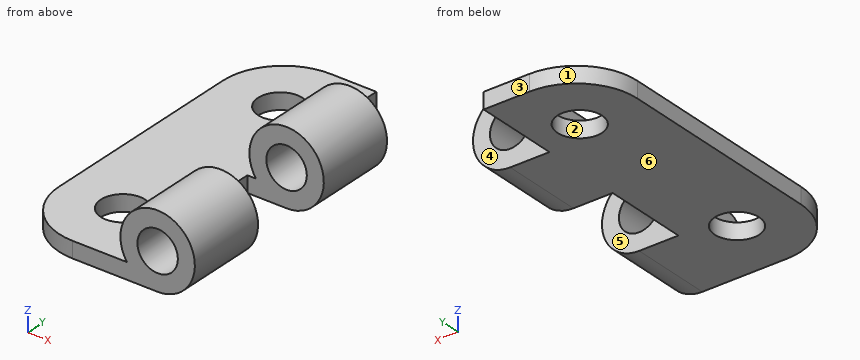
Autodesk Inventor part; units mm, degrees
ref_plane "l_pin_XY" through (0, 0, 0) normal (0, 1, 0) x (1, 0, 0)
ref_plane "l_pin_YZ" through (0, 0, 0) normal (1, 0, 0) x (0, 0, -1)
ref_plane "l_pin_ZX" through (0, 0, 0) normal (0, 0, -1) x (0, 1, 0)
sketch "Sketch_1" plane through (0, 0, 0) normal (0, 0, 1) x (1, 0, 0)
  line L0 (0, -20.5) -> (0, 20.5)
  line L1 (0, 20.5) -> (4.6, 20.5)
  line L2 (4.6, 20.5) -> (4.6, -20.5)
  line L3 (4.6, -20.5) -> (0, -20.5)
  line L4 (0, -20.5) -> (0, 20.5)
revolve "Revolution1" add sketch "Sketch_1" angle 360 about axis through (0, -20.5, 0) along (0, -1, 0)
sketch "Sketch_2" plane through (0, 0, -4.6) normal (0, 0, 1) x (1, 0, 0)
  line L0 (-18, 13) -> (-18, -13)
  arc A0 (-18, -13) -> (-10.5, -20.5) centre (-10.5, -13) ccw
  line L1 (-10.5, -20.5) -> (0, -20.5)
  line L2 (0, -20.5) -> (0, 20.5)
  line L3 (0, 20.5) -> (-10.5, 20.5)
  arc A1 (-10.5, 20.5) -> (-18, 13) centre (-10.5, 13) ccw
extrude "Extrusion1" add sketch "Sketch_2" along normal blind 2
sketch "Sketch_3" plane through (0, 0, 0) normal (0, 0, 1) x (1, 0, 0)
  line L0 (-41, 41) -> (-41, -41)
  line L1 (-41, -41) -> (41, -41)
  line L2 (41, -41) -> (41, 41)
  line L3 (41, 41) -> (-41, 41)
  line L4 (-18, 20.5) -> (-18, -20.5)
  line L5 (-18, -20.5) -> (4.6, -20.5)
  line L6 (4.6, -20.5) -> (4.6, -10.45)
  line L7 (4.6, -10.45) -> (-4.85, -10.45)
  line L8 (-4.85, -10.45) -> (-4.85, 0)
  line L9 (-4.85, 0) -> (4.6, 0)
  line L10 (4.6, 0) -> (4.6, 10.05)
  line L11 (4.6, 10.05) -> (-4.85, 10.05)
  line L12 (-4.85, 10.05) -> (-4.85, 20.5)
  line L13 (-4.85, 20.5) -> (-18, 20.5)
extrude "Extrusion2" cut sketch "Sketch_3" along normal mid plane 82
sketch "Sketch_4" plane through (0, 0, 0) normal (0, 0, 1) x (1, 0, 0)
  line L0 (0, -20.5) -> (0, 20.5)
  line L1 (0, 20.5) -> (2.5, 20.5)
  line L2 (2.5, 20.5) -> (2.5, -20.5)
  line L3 (2.5, -20.5) -> (0, -20.5)
  line L4 (0, -20.5) -> (0, 20.5)
revolve "Revolution2" cut sketch "Sketch_4" angle 360 about axis through (0, -20.5, 0) along (0, -1, 0)
sketch "Sketch_11" plane through (0, 12.5, 0) normal (0, 1, 0) x (1, 0, 0)
  line L0 (-10.5, 2.6) -> (-10.5, 4.6)
  line L1 (-10.5, 4.6) -> (-7.75, 4.6)
  line L2 (-7.75, 4.6) -> (-7.75, 2.6)
  line L3 (-7.75, 2.6) -> (-10.5, 2.6)
  line L4 (-10.5, 2.6) -> (-10.5, 4.6)
revolve "Revolution3" cut sketch "Sketch_11" angle 360 about axis through (-10.5, 12.5, -2.6) along (0, 0, 1)
sketch "Sketch_5" plane through (0, -12.5, 0) normal (0, 1, 0) x (1, 0, 0)
  line L0 (-10.5, 2.6) -> (-10.5, 4.6)
  line L1 (-10.5, 4.6) -> (-7.75, 4.6)
  line L2 (-7.75, 4.6) -> (-7.75, 2.6)
  line L3 (-7.75, 2.6) -> (-10.5, 2.6)
  line L4 (-10.5, 2.6) -> (-10.5, 4.6)
revolve "Revolution4" cut sketch "Sketch_5" angle 360 about axis through (-10.5, -12.5, -2.6) along (0, 0, 1)
ref_plane "l_pin_XY" through (0, 0, 0) normal (0, 1, 0) x (1, 0, 0)
ref_plane "l_pin_YZ" through (0, 0, 0) normal (1, 0, 0) x (0, 0, -1)
ref_plane "l_pin_ZX" through (0, 0, 0) normal (0, 0, -1) x (0, 1, 0)
ref_plane "hole1l_to_bolt_XY" through (-10.5, 12.5, -2.6) normal (0, 0, 1) x (1, 0, 0)
ref_plane "hole1l_to_bolt_YZ" through (-10.5, 12.5, -2.6) normal (1, 0, 0) x (0, 1, 0)
ref_plane "hole1l_to_bolt_ZX" through (-10.5, 12.5, -2.6) normal (0, 1, 0) x (0, 0, 1)
ref_plane "hole2l_to_bolt_XY" through (-10.5, -12.5, -2.6) normal (0, 0, 1) x (1, 0, 0)
ref_plane "hole2l_to_bolt_YZ" through (-10.5, -12.5, -2.6) normal (1, 0, 0) x (0, 1, 0)
ref_plane "hole2l_to_bolt_ZX" through (-10.5, -12.5, -2.6) normal (0, 1, 0) x (0, 0, 1)
ref_plane "hole3l_to_bolt_XY" through (-10.5, 0, -2.6) normal (0, 0, 1) x (1, 0, 0)
ref_plane "hole3l_to_bolt_YZ" through (-10.5, 0, -2.6) normal (1, 0, 0) x (0, 1, 0)
ref_plane "hole3l_to_bolt_ZX" through (-10.5, 0, -2.6) normal (0, 1, 0) x (0, 0, 1)
properties part number "SHHPS5-2-l"
Model file for the job. Use its own axes, mm. Face numbers are marked on the shaded views. A direction names the side the tool comes from. Coordinates: 2 decimals unless noted, no trailing zeros. Write each loop counter-clockwise with the first axis right and the second up, starting at its lowest first coordinate (ties: lowest second). Pieces come first, ordered by that corner, then holes. Notation, with made-up numbers: (46.25, 78) - (104.25, 78) arc R10 ccw to (104.25, 92) - close; hole circle Ø11 at (-33.75, 69.25). An arc over 180 degrees is marked (long way). One line per item, written item: value. Start each with the question number.
1. Slice it at D-D (z = -1.75). Write the cut outline in (x, y).
2. Probe line 1 (Y direction, x = -10.5, z = -3.85); line 2 (Z direction, x = 0, y = -13.5); line 3 (Y direction, x = -2.25, z = 2.5). List the from-to ranges inside material, lowest first. Write a range as from..to.
3. Slice it at A-A (y = 12.5). Write the cut outline in (x, z).
4. Slice it at C-C (x = -12.75). Write the cut outline in (y, z), plus the area to 3 significant figures.
5. Slice it at B-B (y = -12.5). Write the cut outline in (x, z), plus the area to 3 significant figures.
6. Mould opens along X. For the marked faces 1, 2 and 3 say: released by +X, released by -X, zero draft, split by the parting line, or undercut.
7. Flat gauge pins, fed straight in: pin 1 (5 mm diameter, centred on x = 2, y = -3.5, fed in from +Z); pin 2 (11.5 mm diameter, centred on x = -11.5, y = -9.5, fed in from +Z); pin 3 (2 mm diameter, centred on y = 18, z = -4, fed in from +X); pin 4 (4.5 mm diameter, centred on x = 1.5, z = -2, fed in from +Y). Where does each tip first touch, or does it go through?
8. Tool access for the marked faces 4, 5 and 6: list every direction of +Z, -Z, +X, -X, +Y, -Y with a clear straight run to the whole face (end or side of a thin tool).
Answers below:
1. outline: (-4.25, -20.5) - (-1.79, -20.5) - (-1.79, -10.45) - (-4.25, -10.45) - close; (-4.25, 0) - (-1.79, 0) - (-1.79, 10.05) - (-4.25, 10.05) - close; (1.79, -20.5) - (4.25, -20.5) - (4.25, -10.45) - (1.79, -10.45) - close; (1.79, 0) - (4.25, 0) - (4.25, 10.05) - (1.79, 10.05) - close
2. line 1: y = -20.5..-15.25, -9.75..9.75, 15.25..20.5
2. line 2: z = -4.6..-2.5, 2.5..4.6
2. line 3: y = -20.5..-10.45, 0..10.05
3. outline: (-18, -4.6) - (-13.25, -4.6) - (-13.25, -2.6) - (-18, -2.6) - close; (-7.75, -4.6) - (-4.85, -4.6) - (-4.85, -2.6) - (-7.75, -2.6) - close
4. outline: (-20.15, -4.6) - (-14.08, -4.6) - (-14.08, -2.6) - (-20.15, -2.6) - close; (-10.92, -4.6) - (10.92, -4.6) - (10.92, -2.6) - (-10.92, -2.6) - close; (14.08, -4.6) - (20.15, -4.6) - (20.15, -2.6) - (14.08, -2.6) - close
4. area: 68.0 mm^2
5. outline: (-18, -4.6) - (-13.25, -4.6) - (-13.25, -2.6) - (-18, -2.6) - close; (-7.75, -4.6) - (0, -4.6) arc R4.6 ccw (long way) to (-3.79, -2.6) - (-7.75, -2.6) - close; hole circle Ø5 at (0, 0)
5. area: 66.5 mm^2
6. face 1: released by -X
6. face 2: undercut
6. face 3: zero draft
7. pin 1: passes through
7. pin 2: stops at z = -2.6
7. pin 3: stops at x = -4.85
7. pin 4: stops at y = 10.05
8. face 4: +Z, -Z, +X, +Y
8. face 5: +Z, -Z, +X
8. face 6: -Z, +X, -X, +Y, -Y
